Geometry: final body of the model. Coordinates: model frame, mm. Face numbers are marked on the shaded views. A direction names the side the tool comes from. Give positions to 0.01 mm unless a question says otherwise; leave off trailing zeros. Write each loop counter-clockwise with the first axis right and the second up, starting at its lowest first coordinate (ties: lowest second). Pieces come first, ordered by that corner, then holes.
Q1. Section C-C (x = -140.5). Return the cut outline in (y, z).
Q2. Section B-B (y = 176.5). Return the cut outline in (x, z), plus the area to 3 significant figures.
Q3. Mould query, pull axis X, two halves, no side actions, for the marked faces 4, 5 and 6. Classes: +X half, -X half, draft (parallel to the pull), parting line (faces both ways), or undercut.
Q4. Section A-A (z = 119). Return the cut outline in (x, y).
Q5. Line query: line 1 (Z direction, x = 122.5, y = -88.5); line 2 (X direction, y = 50, z = 50); line 3 (X direction, y = 464.5, z = 127). Output: solid intervals per line, ascending.
Q6. Reachability of the marked faces 1, 2 and 3 from +Z, -Z, +X, -X, +Y, -Y: full face, straight path, thin tool, end or side. Return the list, or none.
Q7. Pin query (flat end, axial travel): pin 1 Ø1 at (y, z) = (517, 125) entering from +X (3 decimals); pin 2 Ø10 at (y, z) = (457, 36) entering from -X; pin 3 Ø4 at (x, z) = (151.5, 112.5) entering from -Y; pin 4 Ø10 at (x, y) = (70.5, 487) entering from -Z. Return the tip coordinate at first contact, or that it passes through.
from build123d import *

# Parameters (mm, degrees)
F1_DEPTH      = 127
F3_DEPTH      = 127
F5_DEPTH      = 127
F5_DEPTH_BACK = 127
F6_R          = 72.1706207076
F7_DEPTH      = 266.7


with BuildPart() as f1:
    # F0 (on Top) → F1 (new body)
    with BuildSketch(Plane.XY):
        with BuildLine():
            Line((0, 233.7793111801), (0, 190.5))
            ThreePointArc((0, 190.5), (-164.1023944599, -96.7504735519), (166.6875, -92.2254159316))
            Line((166.6875, -92.2254159316), (254, 0))
            Line((254, 0), (254, 254))
            Line((254, 254), (95.25, 635))
            Line((95.25, 635), (31.75, 635))
            Line((31.75, 635), (31.75, 254))
            Line((31.75, 254), (0, 233.7793111801))
        make_face()
    extrude(amount=F1_DEPTH)

    # F2 (on face) → F3 (join)
    with BuildSketch(Plane.XY.offset(127)):
        with BuildLine():
            ThreePointArc((0, 215.9), (167.9266235199, 135.696201543), (211.0885127336, -45.3260387846))
            Line((211.0885127336, -45.3260387846), (254, 0))
            Line((254, 0), (254, 254))
            Line((254, 254), (95.25, 635))
            Line((95.25, 635), (31.75, 635))
            Line((31.75, 635), (31.75, 254))
            Line((31.75, 254), (0, 233.7793111801))
            Line((0, 233.7793111801), (0, 215.9))
        make_face()
    extrude(amount=F3_DEPTH)

    # F4 (on face) → F5 (join, two sides)
    with BuildSketch(Plane.XY.offset(127)) as f5_sk:
        Polygon((31.75, 539.75), (31.75, 603.25), (-45.7682893979, 571.5), align=None)
        Polygon((31.75, 254.0089488029), (31.75, 285.75), (-49.6154587908, 254), (31.75, 222.25), align=None)
        Polygon((31.75, 285.75), (31.75, 349.25), (-45.7682893979, 317.5), align=None)
        Polygon((31.75, 349.25), (31.75, 412.75), (-45.7682893979, 381), align=None)
        Polygon((31.75, 412.75), (31.75, 476.25), (-45.7682893979, 444.5), align=None)
        Polygon((31.75, 476.25), (31.75, 539.75), (-45.7682893979, 508), align=None)
        Polygon((-45.7682893979, 635), (31.75, 603.25), (31.75, 635), align=None)
    extrude(amount=-F5_DEPTH)
    extrude(f5_sk.sketch, amount=F5_DEPTH_BACK)

    # F6 (on face) → F7 (cut)
    with BuildSketch(Plane.XY.offset(127)):
        Circle(F6_R)
    extrude(amount=-F7_DEPTH, mode=Mode.SUBTRACT)


solid = f1.part
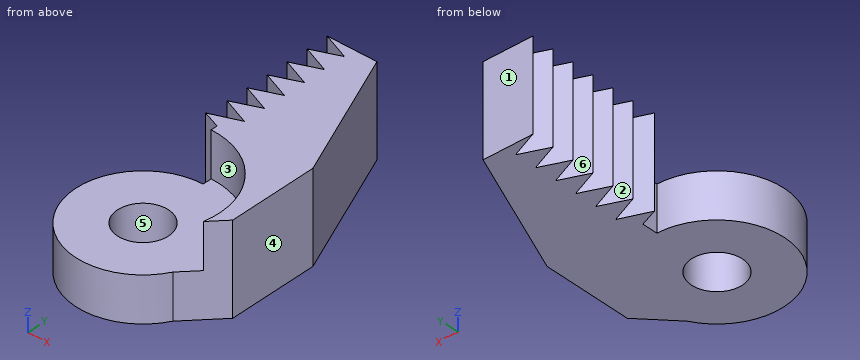
Computed:
1. outline: (-128.65, 0) - (128.65, 0) - (128.65, 127) - (-128.65, 127) - close
2. outline: (-71.68, 0) - (254, 0) - (254, 254) - (124.34, 254) - (124.34, 127) - (-71.68, 127) - close
2. area: 57,800 mm2
3. face 4: +X half
3. face 5: undercut
3. face 6: -X half
4. outline: (-49.62, 254) - (0.84, 234.31) - (0, 233.78) - (0, 190.5) arc R190.5 ccw (long way) to (166.69, -92.23) - (254, 0) - (254, 254) - (95.25, 635) - (-45.77, 635) - (31.75, 603.25) - (-45.77, 571.5) - (31.75, 539.75) - (-45.77, 508) - (31.75, 476.25) - (-45.77, 444.5) - (31.75, 412.75) - (-45.77, 381) - (31.75, 349.25) - (-45.77, 317.5) - (31.75, 285.75) - close; hole circle Ø144.34 at (0, 0)
5. line 1: z = 0 to 127
5. line 2: x = -183.82 to -52.04, 52.04 to 254
5. line 3: x = 3.06 to 166.29
6. face 1: +Z, -Z, +X, -X, +Y
6. face 2: +Z, -Z, -X
6. face 3: +Z, -X
7. pin 1: stops at x = 144.625
7. pin 2: stops at x = -27.46
7. pin 3: stops at y = -118.07
7. pin 4: stops at z = 0
